Autodesk Inventor part; units mm, degrees
ref_plane "YZ Plane" through (0, 0, 0) normal (1, 0, 0) x (0, 1, 0)
ref_plane "XZ Plane" through (0, 0, 0) normal (0, 1, 0) x (-1, 0, 0)
ref_plane "XY Plane" through (0, 0, 0) normal (0, 0, 1) x (1, 0, 0)
sketch "Sketch4" plane through (0, 0, 0) normal (1, 0, 0) x (0, 1, 0)
  line L0 (-25.4, 34.925) -> (-25.4, -34.925)
  line L1 (-25.4, -34.925) -> (0, -34.925)
  line L2 (0, -34.925) -> (0, 34.925)
  line L3 (0, 34.925) -> (-25.4, 34.925)
  line L4 (-25.4, -34.925) -> (-12.7, 0) construction
  line L5 (0, 34.925) -> (50.8, 34.925)
  line L6 (50.8, 34.925) -> (50.8, -34.925)
  line L7 (50.8, -34.925) -> (0, -34.925)
  line L8 (0, -34.925) -> (0, 34.925)
  circle A0 centre (39.6875, 23.8125) radius 4.7625
  circle A1 centre (39.6875, -23.8125) radius 4.7625
  point P0 (0, 0)
  point P1 (-12.7, 0)
  dimension "d2" = 69.85
  dimension "d3" = 25.4
  dimension "d12" = 50.8
  dimension "d15" = 9.525
  dimension "d16" = 11.1125
  dimension "d23" = 11.1125
  dimension "d26" = 11.1125
extrude "Extrusion3" add sketch "Sketch4" along normal mid plane 19.05 contours L3 L2 L1 L0 | L5 L6 L7 L2 | A1
sketch "Sketch6" plane through (-9.525, -25.4, 34.925) normal (0, 0, 1) x (1, 0, 0)
  line L0 (9.525, 25.4) -> (9.525, 0) construction
  line L1 (0, 0) -> (19.05, 0) construction
  line L2 (6.35, 0) -> (12.7, 0)
  line L3 (12.7, 0) -> (12.7, 25.4)
  line L4 (12.7, 25.4) -> (6.35, 25.4)
  line L5 (6.35, 25.4) -> (6.35, 0)
  line L6 (6.35, 0) -> (12.7, 25.4) construction
  line L7 (12.7, 0) -> (6.35, 25.4) construction
  point P0 (9.525, 12.7)
  dimension "d20" = 6.35
extrude "Extrusion4" cut sketch "Sketch6" against normal through all
sketch "Sketch7" plane through (9.525, 0, 0) normal (1, 0, 0) x (0, 0, -1)
  line L0 (34.925, -25.4) -> (34.925, 0)
  line L1 (-34.925, -25.4) -> (34.925, -25.4)
  line L2 (-34.925, 0) -> (-34.925, -25.4)
  line L3 (-34.925, 0) -> (34.925, 0)
  line L4 (-34.925, -85.725) -> (-34.925, -12.7)
  arc A0 (-34.925, -85.725) -> (-22.225, -98.425) centre (-22.225, -85.725) ccw
  line L5 (479.425, -98.425) -> (-22.225, -98.425)
  arc A1 (479.425, -98.425) -> (492.125, -85.725) centre (479.425, -85.725) ccw
  line L6 (492.125, -81.1401) -> (492.125, -85.725)
  arc A2 (492.125, -81.1401) -> (488.7869, -72.5584) centre (479.425, -81.1401) ccw
  line L7 (488.7869, -72.5584) -> (426.0501, -4.1183)
  arc A3 (426.0501, -4.1183) -> (416.6882, 0) centre (416.6882, -12.7) ccw
  line L8 (416.6882, 0) -> (-22.225, 0)
  arc A4 (-22.225, 0) -> (-34.925, -12.7) centre (-22.225, -12.7) ccw
  circle A5 centre (473.075, -79.375) radius 4.826
  circle A6 centre (15.875, -79.375) radius 4.826
  circle A7 centre (457.2, -79.375) radius 4.826
  circle A8 centre (440.1745, -40.6685) radius 3.3782
  circle A9 centre (422.275, -85.725) radius 3.3782
  line L9 (20.6375, -55.8157) -> (20.6375, -25.4)
  arc A10 (23.8125, -22.225) -> (20.6375, -25.4) centre (23.8125, -25.4) ccw
  line L10 (23.8125, -22.225) -> (46.9319, -22.225)
  arc A11 (49.4596, -27.3213) -> (46.9319, -22.225) centre (46.9319, -25.4) ccw
  line L11 (49.4596, -27.3213) -> (26.3402, -57.737)
  arc A12 (20.6375, -55.8157) -> (26.3402, -57.737) centre (23.8125, -55.8157) ccw
  line L12 (28.1443, -71.1037) -> (56.0904, -34.338)
  arc A13 (61.7931, -36.2593) -> (56.0904, -34.338) centre (58.6181, -36.2593) ccw
  line L13 (61.7931, -36.2593) -> (61.7931, -73.025)
  arc A14 (58.6181, -76.2) -> (61.7931, -73.025) centre (58.6181, -73.025) ccw
  line L14 (58.6181, -76.2) -> (30.672, -76.2)
  arc A15 (28.1443, -71.1037) -> (30.672, -76.2) centre (30.672, -73.025) ccw
  line L15 (184.056, -73.025) -> (184.056, -34.8804)
  arc A16 (189.5742, -32.738) -> (184.056, -34.8804) centre (187.231, -34.8804) ccw
  line L16 (189.5742, -32.738) -> (224.451, -70.8826)
  arc A17 (222.1078, -76.2) -> (224.451, -70.8826) centre (222.1078, -73.025) ccw
  line L17 (222.1078, -76.2) -> (187.231, -76.2)
  arc A18 (184.056, -73.025) -> (187.231, -76.2) centre (187.231, -73.025) ccw
  line L18 (291.2199, -27.5424) -> (254.7557, -67.4233)
  arc A19 (249.2375, -65.2808) -> (254.7557, -67.4233) centre (252.4125, -65.2808) ccw
  line L19 (249.2375, -65.2808) -> (249.2375, -25.4)
  arc A20 (252.4125, -22.225) -> (249.2375, -25.4) centre (252.4125, -25.4) ccw
  line L20 (252.4125, -22.225) -> (288.8767, -22.225)
  arc A21 (291.2199, -27.5424) -> (288.8767, -22.225) centre (288.8767, -25.4) ccw
  line L21 (234.1943, -67.4233) -> (197.7301, -27.5424)
  arc A22 (200.0733, -22.225) -> (197.7301, -27.5424) centre (200.0733, -25.4) ccw
  line L22 (200.0733, -22.225) -> (236.5375, -22.225)
  arc A23 (239.7125, -25.4) -> (236.5375, -22.225) centre (236.5375, -25.4) ccw
  line L23 (239.7125, -25.4) -> (239.7125, -65.2808)
  arc A24 (234.1943, -67.4233) -> (239.7125, -65.2808) centre (236.5375, -65.2808) ccw
  line L24 (304.894, -34.8804) -> (304.894, -73.025)
  arc A25 (301.719, -76.2) -> (304.894, -73.025) centre (301.719, -73.025) ccw
  line L25 (301.719, -76.2) -> (266.8422, -76.2)
  arc A26 (264.499, -70.8826) -> (266.8422, -76.2) centre (266.8422, -73.025) ccw
  line L26 (264.499, -70.8826) -> (299.3758, -32.738)
  arc A27 (304.894, -34.8804) -> (299.3758, -32.738) centre (301.719, -34.8804) ccw
  line L27 (341.3125, -25.4) -> (341.3125, -73.025)
  arc A28 (338.1375, -76.2) -> (341.3125, -73.025) centre (338.1375, -73.025) ccw
  line L28 (338.1375, -76.2) -> (317.594, -76.2)
  arc A29 (314.419, -73.025) -> (317.594, -76.2) centre (317.594, -73.025) ccw
  line L29 (314.419, -73.025) -> (314.419, -25.4)
  arc A30 (317.594, -22.225) -> (314.419, -25.4) centre (317.594, -25.4) ccw
  line L30 (317.594, -22.225) -> (338.1375, -22.225)
  arc A31 (341.3125, -25.4) -> (338.1375, -22.225) centre (338.1375, -25.4) ccw
  line L31 (400.05, -69.85) -> (400.05, -29.1831)
  arc A32 (405.5794, -27.053) -> (400.05, -29.1831) centre (403.225, -29.1831) ccw
  line L32 (405.5794, -27.053) -> (445.2458, -70.8949)
  arc A33 (442.8915, -76.2) -> (445.2458, -70.8949) centre (442.8915, -73.025) ccw
  line L33 (442.8915, -76.2) -> (406.4, -76.2)
  arc A34 (400.05, -69.85) -> (406.4, -76.2) centre (406.4, -69.85) ccw
  circle A35 centre (83.3958, -57.6072) radius 5.5626
  circle A36 centre (160.8658, -32.2072) radius 5.5626
  circle A37 centre (83.3958, -32.2072) radius 5.5626
  circle A38 centre (160.8658, -57.6072) radius 5.5626
  circle A39 centre (358.775, -28.575) radius 2.5527
  circle A40 centre (368.3, -19.05) radius 2.5527
  circle A41 centre (377.825, -9.525) radius 2.5527
  circle A42 centre (358.775, -88.9) radius 2.5527
  circle A43 centre (377.825, -69.85) radius 2.5527
  circle A44 centre (368.3, -79.375) radius 2.5527
  circle A45 centre (-9.525, -12.7) radius 3.3782
  circle A46 centre (-9.525, -85.725) radius 3.3782
  circle A47 centre (15.875, -12.7) radius 3.3782
  circle A48 centre (41.275, -12.7) radius 3.3782
  circle A49 centre (41.275, -85.725) radius 3.3782
  circle A50 centre (66.675, -12.7) radius 3.3782
  circle A51 centre (92.075, -12.7) radius 3.3782
  circle A52 centre (92.075, -85.725) radius 3.3782
  circle A53 centre (117.475, -12.7) radius 3.3782
  circle A54 centre (117.475, -85.725) radius 3.3782
  circle A55 centre (142.875, -12.7) radius 3.3782
  circle A56 centre (142.875, -85.725) radius 3.3782
  circle A57 centre (168.275, -12.7) radius 3.3782
  circle A58 centre (193.675, -12.7) radius 3.3782
  circle A59 centre (193.675, -85.725) radius 3.3782
  circle A60 centre (219.075, -12.7) radius 3.3782
  circle A61 centre (219.075, -85.725) radius 3.3782
  circle A62 centre (244.475, -12.7) radius 3.3782
  circle A63 centre (269.875, -12.7) radius 3.3782
  circle A64 centre (269.875, -85.725) radius 3.3782
  circle A65 centre (295.275, -12.7) radius 3.3782
  circle A66 centre (295.275, -85.725) radius 3.3782
  circle A67 centre (320.675, -12.7) radius 3.3782
  circle A68 centre (320.675, -85.725) radius 3.3782
  circle A69 centre (346.075, -12.7) radius 3.3782
  circle A70 centre (346.075, -85.725) radius 3.3782
  circle A71 centre (396.875, -12.7) radius 3.3782
  circle A72 centre (396.875, -85.725) radius 3.3782
  circle A73 centre (419.1, -15.875) radius 4.953
  circle A74 centre (66.5556, -90.5002) radius 3.3528
  circle A75 centre (177.706, -90.5002) radius 3.3528
  circle A76 centre (122.1308, -60.325) radius 14.2812
  circle A77 centre (244.475, -83.185) radius 4.826
  circle A78 centre (-9.525, -12.7) radius 3.3782
  circle A79 centre (15.875, -12.7) radius 3.3782
  point P0 (0, 0)
extrude "Extrusion5" cut sketch "Sketch7" against normal through all contours A45 | A47
sketch "Sketch8" plane through (9.525, 0, 0) normal (1, 0, 0) x (0, 0, -1)
  circle A0 centre (-23.8125, 39.6875) radius 4.7625
  circle A1 centre (23.8125, 39.6875) radius 4.7625
  line L0 (34.925, -25.4) -> (34.925, 50.8)
  point P0 (0, 0)
  dimension "d27" = 11.1125
extrude "Extrusion6" cut sketch "Sketch8" against normal through all contours A1
properties part number "NarrowSupportForLift" material "Aluminum 6061"
The listing builds one solid part. Answer for the finished solid, in the listing's coordinates (mm). A direction names the side the tool comes from. Give positions to 0.01 mm unless a question says otherwise; leave off trailing zeros. Loops run counter-clockwise (first coordinate to the right, second up) from the corner with the lowest first, then second, coordinate; pieces in that order, holes last.
Item 1: A cutting plane is placed at C-C (y = -12.7). Give the vertices of the cut face in (x, z) (3 decimals), then the cut area to 3 significant figures.
Derived:
outline: (-9.525, -34.925) - (-3.175, -34.925) - (-3.175, -19.253) - (-9.525, -19.253) - close; (-9.525, -12.497) - (-3.175, -12.497) - (-3.175, 6.147) - (-9.525, 6.147) - close; (-9.525, 12.903) - (-3.175, 12.903) - (-3.175, 34.925) - (-9.525, 34.925) - close; (3.175, -34.925) - (9.525, -34.925) - (9.525, -19.253) - (3.175, -19.253) - close; (3.175, -12.497) - (9.525, -12.497) - (9.525, 6.147) - (3.175, 6.147) - close; (3.175, 12.903) - (9.525, 12.903) - (9.525, 34.925) - (3.175, 34.925) - close
area: 715 mm2
Item 2: A cutting plane is placed at D-D (z = -13.5). Give the vertices of the cut face in (x, y) (3 decimals), then the cut area to 3 significant figures.
Derived:
outline: (-9.525, -25.4) - (-3.175, -25.4) - (-3.175, -15.102) - (-9.525, -15.102) - close; (-9.525, -10.298) - (-3.175, -10.298) - (-3.175, 0) - (3.175, 0) - (3.175, -10.298) - (9.525, -10.298) - (9.525, 50.8) - (-9.525, 50.8) - close; (3.175, -25.4) - (9.525, -25.4) - (9.525, -15.102) - (3.175, -15.102) - close
area: 1,230 mm2
Item 3: A cutting plane is placed at A-A (y = -2). Give the vertices of the cut face in (x, z) (3 decimals).
Derived:
outline: (-9.525, -34.925) - (-3.175, -34.925) - (-3.175, 34.925) - (-9.525, 34.925) - close; (3.175, -34.925) - (9.525, -34.925) - (9.525, 34.925) - (3.175, 34.925) - close
Item 4: Each of these flat-tipped pins is pushed along its axis until it touches: pin 1 Ø6 at (y, z) = (-12.7, 9.525) entering from +X; pin 2 Ø4 at (x, z) = (1, -0.5) entering from -Y. Where does it stop, or does it pass through?
Derived:
pin 1: passes through
pin 2: stops at y = 0
Item 5: A tool of negligible diameter and unlimited length cuts with its end or side. For faces 1 (the flat face through (-6, -25.4, 0)), 2 (the flat face through (-3.175, -13, 0)), from which of +Z, -Z, +X, -X, +Y, -Y can it reach the whole face along a straight path? Write none if from no direction.
Derived:
face 1: +Z, -Z, +X, -X, -Y
face 2: +Z, -Z, -Y
Item 6: A cutting plane is placed at B-B (z = 27). Give the vertices of the cut face in (x, y) (3 decimals), then the cut area to 3 significant figures.
Derived:
outline: (-9.525, -25.4) - (-3.175, -25.4) - (-3.175, 0) - (3.175, 0) - (3.175, -25.4) - (9.525, -25.4) - (9.525, 36.149) - (-9.525, 36.149) - close; (-9.525, 43.226) - (9.525, 43.226) - (9.525, 50.8) - (-9.525, 50.8) - close
area: 1,160 mm2
Item 7: Determine the mould class of faces 3 (the flat face through (0, 13, 34.925)), 4 (the cylindrical face through (-0.133, 38.655, 28.462)), 5 (the flat face through (3.175, -13, 0)) for opening direction Z: +Z half, -Z half, draft (parallel to the pull), parting line (faces both ways), or undercut.
Derived:
face 3: +Z half
face 4: undercut
face 5: draft
Item 8: Find the intervals of material crossed by line 1 along X through (y, z) = (-5, 29) (3 decimals); line 2 along Z through (x, y) = (0.75, 41.5) (3 decimals); line 3 along Z through (x, y) = (5, 43) (3 decimals), in increasing order.
Derived:
line 1: x = -9.525 to -3.175, 3.175 to 9.525
line 2: z = -34.925 to -28.217, -19.408 to 19.408, 28.217 to 34.925
line 3: z = -34.925 to -27.234, -20.391 to 20.391, 27.234 to 34.925
